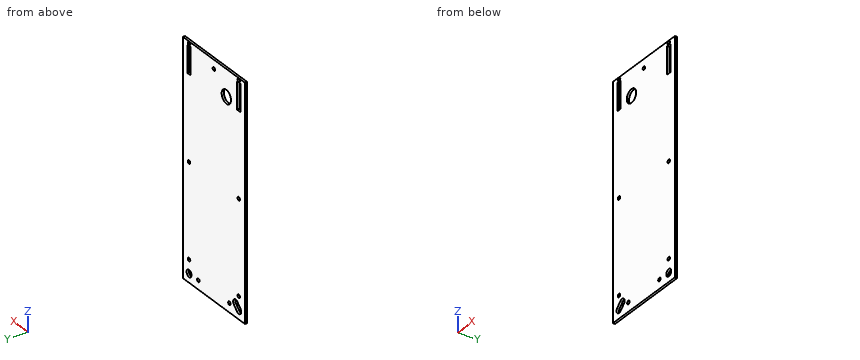
from build123d import *

# Parameters (mm, degrees)
SKETCH1_W           = 127
SKETCH1_H           = 330.2
BOSS_EXTRUDE1_DEPTH = 3.175
SKETCH2_R           = 5.08
SKETCH2_R_2         = 2.5
CUT_EXTRUDE1_DEPTH  = 25.4
SKETCH3_R           = 2.5
SKETCH3_R_2         = 9.525
CUT_EXTRUDE2_DEPTH  = 25.4


with BuildPart() as part:
    # Sketch1 → Boss-Extrude1 (new body)
    with BuildSketch(Plane(origin=(0, 0, 0), x_dir=(1, 0, 0), z_dir=(0, 1, 0))):
        Rectangle(SKETCH1_W, SKETCH1_H)
    extrude(amount=BOSS_EXTRUDE1_DEPTH)

    # Sketch2 → Cut-Extrude1 (cut)
    with BuildSketch(Plane(origin=(0, 3.175, 0), x_dir=(1, 0, 0), z_dir=(0, 1, 0))):
        with Locations((50.8, 152.4)):
            Circle(SKETCH2_R)
        with Locations((-31.75, 152.4)):
            Circle(SKETCH2_R_2)
        with Locations((31.75, 152.4)):
            Circle(SKETCH2_R_2)
        with Locations((-50.8, 133.35)):
            Circle(SKETCH2_R_2)
        with Locations((50.8, 133.35)):
            Circle(SKETCH2_R_2)
        with Locations((-50.8, -161.925)):
            Circle(SKETCH2_R_2)
        with Locations((50.8, -161.925)):
            Circle(SKETCH2_R_2)
        with Locations((-50.8, 0)):
            Circle(SKETCH2_R_2)
        with Locations((50.8, 0)):
            Circle(SKETCH2_R_2)
        with Locations((0, -152.4)):
            Circle(SKETCH2_R_2)
        with BuildLine():
            Line((-54.392102448, 148.807897552), (-48.042102448, 142.457897552))
            ThreePointArc((-48.042102448, 142.457897552), (-40.857897552, 142.457897552), (-40.857897552, 149.642102448))
            Line((-40.857897552, 149.642102448), (-47.207897552, 155.992102448))
            ThreePointArc((-47.207897552, 155.992102448), (-54.392102448, 155.992102448), (-54.392102448, 148.807897552))
        make_face()
    extrude(amount=-CUT_EXTRUDE1_DEPTH, mode=Mode.SUBTRACT)

    # Sketch3 → Cut-Extrude2 (cut)
    with BuildSketch(Plane(origin=(0, 3.175, 0), x_dir=(1, 0, 0), z_dir=(0, 1, 0))):
        with Locations((-50.8, -161.925)):
            Circle(SKETCH3_R)
        Polygon((-54.3, -127.2), (-54.3, -120.2), (-47.3, -120.2), (-47.3, -127.2), (-47.3, -152.2), (-47.3, -159.2), (-54.3, -159.2), (-54.3, -152.2), align=None)
        with Locations((-25.4, -127)):
            Circle(SKETCH3_R_2)
        Polygon((54.3, -127.2), (54.3, -152.2), (54.3, -159.2), (47.3, -159.2), (47.3, -152.2), (47.3, -127.2), (47.3, -120.2), (54.3, -120.2), align=None)
    extrude(amount=-CUT_EXTRUDE2_DEPTH, mode=Mode.SUBTRACT)


solid = part.part
Geometry check sheet. Reference: the model listing, model coordinates, mm. Give positions to 0.01 mm unless a question says otherwise; leave off trailing zeros. Loops run counter-clockwise (first coordinate to the right, second up) from the corner with the lowest first, then second, coordinate; pieces in that order, holes last. Notation, with made-up numbers: M -21,40 L 28,40 A6 cw 28,50 Z; hole C 22,88.25 d10. An arc over 180 degrees is marked long. Answer as a JSON object with one key per item and string values. Group by question number.
Item 1: Sectioned sample at B-B on x = -23.5. Record the boundary of the cut face in (y, z) (3 decimals).
Item 2: Sectioned sample at C-C on y = 0.5. Give the number of separate pieces and of enclosed holes in the cut face, plus the area to 3 significant figures.
Item 3: Material ranges on L1, parallel to X at y = 1.6, z = 0; L2, parallel to Z at x = 50.8, y = 1.3 (3 decimals); L3, parallel to Z at x = -25.4, y = 0.9 (3 decimals), recorded low to high.
Item 4: Sectioned sample at A-A on z = 133. Record the boundary of the cut face in (x, y) (3 decimals).
Item 5: Gauge pin test, flat ends, axial feed: pin 1 (11.5 mm diameter, centred on x = -25.4, z = 127, fed in from +Y); pin 2 (8 mm diameter, centred on x = -50.8, z = -133.35, fed in from -Y). Record the tip position at first contact, or that the pin passes through.
Findings below:
{
 "1": {"outline": "M 0,-165.1 L 3.175,-165.1 L 3.175,117.666 L 0,117.666 Z; M 0,136.334 L 3.175,136.334 L 3.175,165.1 L 0,165.1 Z"},
 "2": {"separate pieces": "1", "enclosed holes": "14", "area": "40,700 mm2"},
 "3": {"L1": "-63.5 to -53.3, -48.3 to 48.3, 53.3 to 63.5", "L2": "-165.1 to -157.48, -147.32 to -135.85, -130.85 to -2.5, 2.5 to 120.2, 159.2 to 159.425, 164.425 to 165.1", "L3": "-165.1 to 117.475, 136.525 to 165.1"},
 "4": {"outline": "M -63.5,0 L -54.3,0 L -54.3,3.175 L -63.5,3.175 Z; M -47.3,0 L -32.798,0 L -32.798,3.175 L -47.3,3.175 Z; M -18.002,0 L 47.3,0 L 47.3,3.175 L -18.002,3.175 Z; M 54.3,0 L 63.5,0 L 63.5,3.175 L 54.3,3.175 Z"},
 "5": {"pin 1": "through", "pin 2": "y = 0"}
}
